The listing builds one solid part. Answer for the finished solid, in the listing's coordinates (mm). Face numbers are marked on the shaded views. A direction names the side the tool comes from. Round coordinates to 2 decimals unless told otherwise and drop trailing zeros. Loops run counter-clockwise (first coordinate to the right, second up) from the corner with the lowest first, then second, coordinate; pieces in that order, holes last. Notation, with made-up numbers: M 25,-10.5 L 29,-10.5 A29 ccw 29,10.5 Z; hole C 29.25,-18 d3. An arc over 180 degrees is marked long. Put each result on its own line as item: value. Start each with the question number.
(1) Determine the mould class of the marked faces 4, 5, 6 and 7 for opening direction Z: released by +Z, released by -Z, zero draft, split by the parting line, or undercut.
(2) Straight lines are drawn through the part: line 1 (Z direction, x = -13, y = 14); line 2 (X direction, y = 3, z = -16); line 3 (X direction, y = 9.5, z = 3). For each, find the intervals that lie inside material, in ascending order.
(3) Which of the six approach directions +Z, -Z, +X, -X, +Y, -Y give full straight-line access (tool end or side, diameter ignored) to the marked faces 1, 2 and 3?
(4) Section B-B, the plane z = 8 is taken. Determine the outline of the cut face in (x, y).
(5) Flat-ended cylindrical pins translate along their axes: P1, Ø3, axis at x = -42.5, y = 11, coming from the +Z side; P2, Ø4, axis at x = 10.5, y = 21.5, coming from the +Z side; P3, Ø1.2, axis at x = -40.5, y = 4, coming from the +Z side. Find the tip coordinate at first contact, or state that the pin passes through.
(6) Section D-D, the plane y = 29 is taken. Determine the outline of the cut face in (x, z).
(7) Section C-C, the plane y = 7 is taken. Determine the outline of the cut face in (x, z), then the cut area to 3 significant figures.
(8) Section A-A, the plane x = -22 is taken. Determine the outline of the cut face in (y, z).
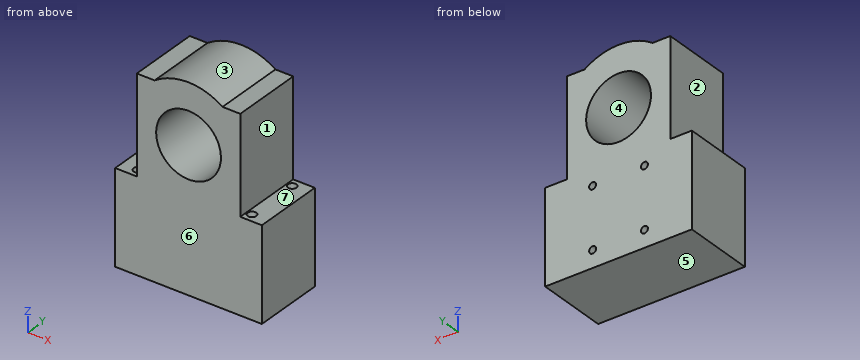
```python
from build123d import *

# Parameters (mm, degrees)
SKETCH1_R           = 15
BOSS_EXTRUDE3_DEPTH = 33
SKETCH12_R          = 2
CUT_EXTRUDE1_DEPTH  = 10
SKETCH13_W          = 67.899494937
SKETCH13_H          = 35
BOSS_EXTRUDE4_DEPTH = 33
SKETCH14_R          = 1.62
CUT_EXTRUDE2_DEPTH  = 10


with BuildPart() as part:
    # Sketch1 → Boss-Extrude3 (new body)
    with BuildSketch(Plane(origin=(0, 0, 0), x_dir=(1, 0, 0), z_dir=(0, 1, 0))):
        with BuildLine():
            Line((-47.308295415, 17.815966111), (20.591199522, 17.815966111))
            Line((20.591199522, 17.815966111), (20.591199522, 9.675262593))
            Line((20.591199522, 9.675262593), (10.591199522, 9.675262593))
            Line((10.591199522, 9.675262593), (10.591199522, -35.324737407))
            Line((10.591199522, -35.324737407), (2.365275891, -35.324737407))
            ThreePointArc((2.365275891, -35.324737407), (-13.358547947, -40.274484875), (-29.082371784, -35.324737407))
            Line((-29.082371784, -35.324737407), (-37.308295415, -35.324737407))
            Line((-37.308295415, -35.324737407), (-37.308295415, 9.675262593))
            Line((-37.308295415, 9.675262593), (-47.308295415, 9.675262593))
            Line((-47.308295415, 9.675262593), (-47.308295415, 17.815966111))
        make_face()
        with Locations(Location((-13.358547947, -12.824737407, 0), (0, 0, 270))):
            Circle(SKETCH1_R, mode=Mode.SUBTRACT)
    extrude(amount=BOSS_EXTRUDE3_DEPTH)

    # Sketch12 → Cut-Extrude1 (cut)
    with BuildSketch(Plane(origin=(0, 0, -17.815966111), x_dir=(-1, 0, 0), z_dir=(0, 0, -1))):
        with Locations((39.788295415, 4)):
            Circle(SKETCH12_R)
        with Locations((39.788295415, 29)):
            Circle(SKETCH12_R)
        with Locations((-13.071199522, 29)):
            Circle(SKETCH12_R)
        with Locations((-13.071199522, 4)):
            Circle(SKETCH12_R)
    extrude(amount=-CUT_EXTRUDE1_DEPTH, mode=Mode.SUBTRACT)

    # Sketch13 → Boss-Extrude4 (add)
    with BuildSketch(Plane(origin=(0, 33, 0), x_dir=(1, 0, 0), z_dir=(0, 1, 0))):
        with Locations((-13.358547947, 35.315966111)):
            Rectangle(SKETCH13_W, SKETCH13_H)
    extrude(amount=-BOSS_EXTRUDE4_DEPTH)

    # Sketch14 → Cut-Extrude2 (cut)
    with BuildSketch(Plane(origin=(0, 33, 0), x_dir=(1, 0, 0), z_dir=(0, 1, 0))):
        with Locations(Location((-25.358295415, 16.899970921, 0), (0, 0, 270))):
            Circle(SKETCH14_R)
        with Locations(Location((-1.358295415, 16.899970921, 0), (0, 0, 270))):
            Circle(SKETCH14_R)
        with Locations(Location((-25.358295415, 44.899970921, 0), (0, 0, 270))):
            Circle(SKETCH14_R)
        with Locations(Location((-1.358295415, 44.899970921, 0), (0, 0, 270))):
            Circle(SKETCH14_R)
    extrude(amount=-CUT_EXTRUDE2_DEPTH, mode=Mode.SUBTRACT)


solid = part.part
```
Recorded:
1. face 4: undercut
1. face 5: released by -Z
1. face 6: zero draft
1. face 7: released by +Z
2. line 1: z = -52.82 to -2.17, 27.82 to 40.27
2. line 2: x = -47.31 to -41.52, -38.06 to 11.34, 14.8 to 20.59
2. line 3: x = -37.31 to -24.69, -2.02 to 10.59
3. face 1: +Z, +X, +Y, -Y
3. face 2: +Z, -X, +Y, -Y
3. face 3: +Z, +Y, -Y
4. outline: M -37.31,0 L -27.56,0 L -27.56,33 L -37.31,33 Z; M 0.84,0 L 10.59,0 L 10.59,33 L 0.84,33 Z
5. P1: stops at z = -9.68
5. P2: stops at z = 35.32
5. P3: stops at z = -17.82
6. outline: M -47.31,-52.82 L 20.59,-52.82 L 20.59,-9.68 L 15.07,-9.68 L 15.07,-17.82 L 11.07,-17.82 L 11.07,-9.68 L 10.59,-9.68 L 10.59,35.32 L 2.37,35.32 A27.45 ccw -29.08,35.32 L -37.31,35.32 L -37.31,-9.68 L -37.79,-9.68 L -37.79,-17.82 L -41.79,-17.82 L -41.79,-9.68 L -47.31,-9.68 Z; hole C -13.36,12.82 d30; hole C -25.36,-44.9 d3.24; hole C -25.36,-16.9 d3.24; hole C -1.36,-44.9 d3.24; hole C -1.36,-16.9 d3.24
7. outline: M -47.31,-52.82 L 20.59,-52.82 L 20.59,-9.68 L 10.59,-9.68 L 10.59,35.32 L 2.37,35.32 A27.45 ccw -29.08,35.32 L -37.31,35.32 L -37.31,-9.68 L -47.31,-9.68 Z; hole C -13.36,12.82 d30
7. area: 4,480 mm²
8. outline: M 0,-52.82 L 33,-52.82 L 33,0.56 L 0,0.56 Z; M 0,25.09 L 33,25.09 L 33,38.88 L 0,38.88 Z
